Design review of the part shown in the three views and the two pictorial views. Dimensions are in mm from the part's minimum x, y and z. A direction names the side the tool comes from. Coordinates: 2 decimals unless noted, no trailing zeros. Write each loop counter-clockwise with the first axis right and the second up, starting at its lowest first coordinate (ties: lowest second). Pieces come first, ordered by that corner, then holes. Notation, with made-up numbers: M 48,20 L 96,20 A20 cw 96,33 Z; hole C 61.5,22 d3. An arc over 180 degrees is marked long. Answer as a JSON object with one key per item and string values.
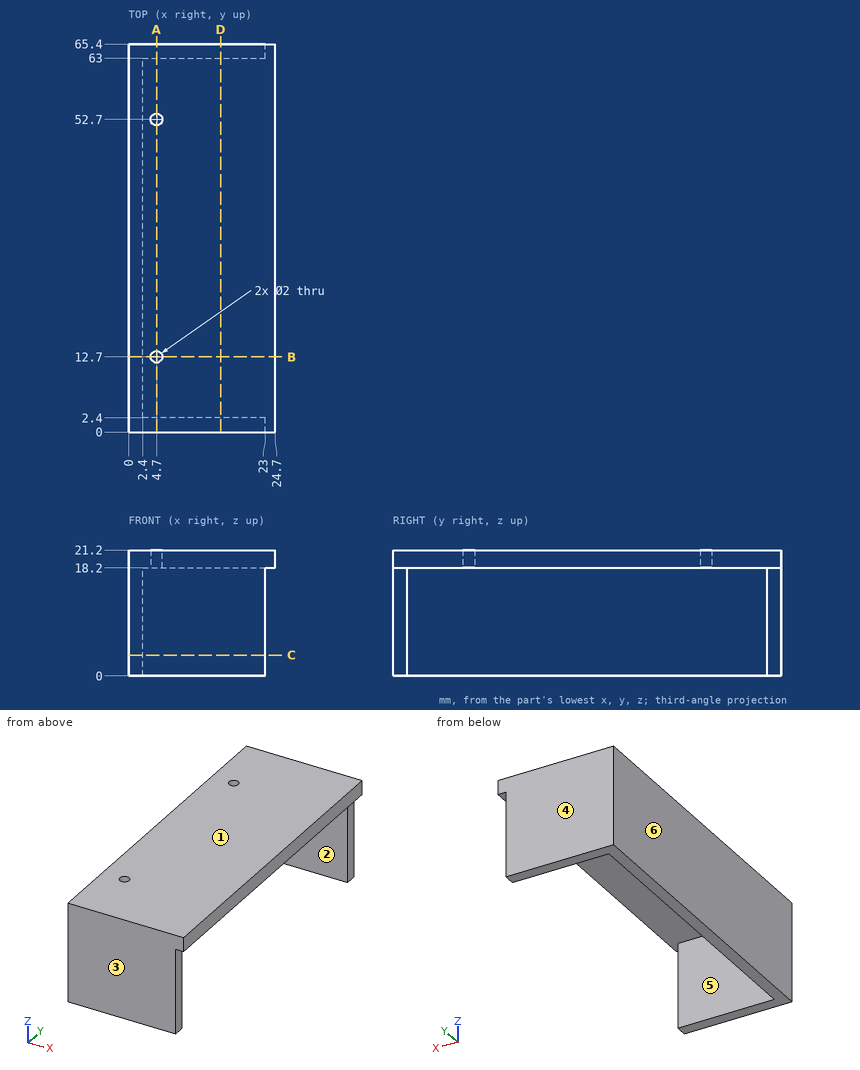
(1) Add section A-A on x = 4.7. Give the boundary of the cut face in (y, z), and give its area (3 significant figures).
Results list:
{"outline": "M 0,0 L 2.4,0 L 2.4,18.2 L 11.7,18.2 L 11.7,21.2 L 0,21.2 Z; M 13.7,18.2 L 51.7,18.2 L 51.7,21.2 L 13.7,21.2 Z; M 53.7,18.2 L 63,18.2 L 63,0 L 65.4,0 L 65.4,21.2 L 53.7,21.2 Z", "area": "272 mm²"}
(2) Wall thickness on line 1 along Y through (x, z) = (4.7, 19.65); line 2 along Y through (x, z) = (22, 3.25); line 3 along X through (y, z) = (52.7, 20.55): over which ranges is each line inside the solid? List them lowest first. Write a range as from..to.
Results list:
{"line 1": "0..11.7, 13.7..51.7, 53.7..65.4", "line 2": "0..2.4, 63..65.4", "line 3": "0..3.7, 5.7..24.7"}
(3) For pin 1 Ø1.9 at (y, z) = (1.5, 6.5) entering from +X; pin 2 Ø3 at (x, y) = (4.7, 12.7) entering from -Z, all flat-tipped, find the tip position at first contact; note any pin that passes through.
Results list:
{"pin 1": "x = 23", "pin 2": "z = 18.2"}
(4) Add section D-D on x = 15.5. Give the boundary of the cut face in (y, z), and give its area (3 significant figures).
Results list:
{"outline": "M 0,0 L 2.4,0 L 2.4,18.2 L 63,18.2 L 63,0 L 65.4,0 L 65.4,21.2 L 0,21.2 Z", "area": "284 mm²"}
(5) For the marked faces 1 and 2, list the 3-axis set-ups (+Z, -Z, +X, -X, +Y, -Y) from which the entire face can be reached by the end or side of a thin tool; tool diameter is ignored.
Results list:
{"face 1": "+Z, +X, -X, +Y, -Y", "face 2": "-Z, +X"}
(6) Add section C-C on z = 3.5. Give the boundary of the cut face in (x, y), and give its area (3 significant figures).
Results list:
{"outline": "M 0,0 L 23,0 L 23,2.4 L 2.4,2.4 L 2.4,63 L 23,63 L 23,65.4 L 0,65.4 Z", "area": "256 mm²"}
(7) Draft analysis for pull direction Y (two halves, no side actions). For the marked faces 3, 4, 5 and 6, state which applies: released by +Y, released by -Y, zero draft, split by the parting line, or undercut.
Results list:
{"face 3": "released by -Y", "face 4": "released by +Y", "face 5": "undercut", "face 6": "zero draft"}
(8) Add section B-B on y = 12.7. Give the boundary of the cut face in (x, z).
Results list:
{"outline": "M 0,0 L 2.4,0 L 2.4,18.2 L 3.7,18.2 L 3.7,21.2 L 0,21.2 Z; M 5.7,18.2 L 24.7,18.2 L 24.7,21.2 L 5.7,21.2 Z"}
